Build history of the part. All positions in model axes, mm. Face numbers are marked on the shaded views. Give positions to 0.01 mm unless a question says otherwise; leave off trailing zeros. Order: outer loops, then holes, each group sorted by start corner. A loop starts at its lowest first (then second) coordinate and runs counter-clockwise, first axis right, second up. Notation, with made-up numbers: (10, -26) - (20, -26) arc R8 cw to (20, -11) - close; hole circle Ø3 at (28, 61). An arc over 180 degrees is marked (long way). One line per item, written item: value.
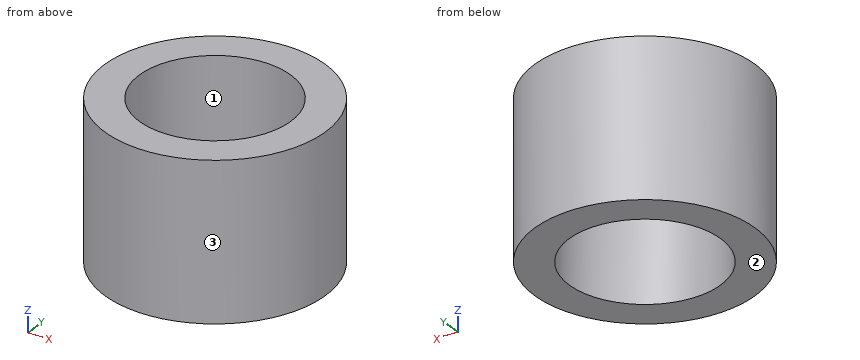
```python
from build123d import *

# Parameters (mm, degrees)
F0_R     = 35.413453
F1_DEPTH = 50
F2_R     = 30.967597
F3_DEPTH = 50
F4_R     = 30.405433
F5_DEPTH = 50
F6_R     = 24.310595
F7_DEPTH = 50


with BuildPart() as f1:
    # F0 (on Top) → F1 (new body)
    with BuildSketch(Plane.XY):
        Circle(F0_R)
    extrude(amount=F1_DEPTH)

    # F2 (on Top) → F3 (cut)
    with BuildSketch(Plane.XY):
        Circle(F2_R)
    extrude(amount=-F3_DEPTH, mode=Mode.SUBTRACT)

    # F4 (on Top) → F5 (cut)
    with BuildSketch(Plane.XY):
        Circle(F4_R)
    extrude(amount=-F5_DEPTH, mode=Mode.SUBTRACT)

    # F6 (on Top) → F7 (cut)
    with BuildSketch(Plane.XY):
        Circle(F6_R)
    extrude(amount=F7_DEPTH, mode=Mode.SUBTRACT)


solid = f1.part
```
(1) Slice it at C-C, the plane z = 11.5. Give the cut face in (x, y), and give its area (3 significant figures).
Completed:
outline: circle Ø70.83 at (0, 0); hole circle Ø48.62 at (0, 0)
area: 2,080 mm²
(2) Pin check, flat tips, straight feed: P1, Ø1, axis at y = -24.5, z = 14.5, coming from the -X side; P2, Ø5, axis at y = -23, z = 26.5, coming from the +X side; P3, Ø1, axis at y = -4, z = 9.5, coming from the +X side. Stop position of each tip, or through.
Completed:
P1: x = -26.04
P2: x = 28.88
P3: x = 35.24
(3) Drill centre lines: line 1 (Y direction, x = 0, z = 17); line 2 (X direction, y = 5, z = 29); line 3 (X direction, y = 19, z = 45) (3 decimals). Where is each one in solid material? Low to high.
Completed:
line 1: -35.41 to -24.31, 24.31 to 35.41
line 2: -35.06 to -23.79, 23.79 to 35.06
line 3: -29.885 to -15.166, 15.166 to 29.885
(4) Slice it at A-A, the plane x = 0. Give the cut face in (y, z).
Completed:
outline: (-35.41, 0) - (-24.31, 0) - (-24.31, 50) - (-35.41, 50) - close; (24.31, 0) - (35.41, 0) - (35.41, 50) - (24.31, 50) - close
(5) Pull direction Y, two halves, no side cores. Call the marked faces 1, 2 and 3: +Y half, -Y half, draft (parallel to the pull), parting line (faces both ways), or undercut.
Completed:
face 1: undercut
face 2: draft
face 3: parting line
(6) Slice it at D-D, the plane x = -30. Give the cut face in (y, z).
Completed:
outline: (-18.82, 0) - (18.82, 0) - (18.82, 50) - (-18.82, 50) - close
